from build123d import *

# Parameters (mm, degrees)
SKETCH1_R           = 9.2
BOSS_EXTRUDE1_DEPTH = 8.2
BOSS_EXTRUDE2_DEPTH = 1.8
LPATTERN1_COUNT     = 3
LPATTERN1_PITCH     = 20.2
FILLET1_R           = 1
CUT_EXTRUDE1_DEPTH  = 8.2


with BuildPart() as part:
    # Sketch1 → Boss-Extrude1 (new body)
    with BuildSketch(Plane(origin=(0, 0, 0), x_dir=(1, 0, 0), z_dir=(0, 1, 0))):
        Polygon((-9.1, 10.1), (-7, 10.1), (-7.5, 8.7), (-4.5, 8.7), (-5, 10.1), (5, 10.1), (4.5, 8.7), (7.5, 8.7), (7, 10.1), (9.1, 10.1), (10.1, 10.1), (10.1, 9.1), (10.1, 7), (10.1, 5), (10.1, -5), (10.1, -7), (10.1, -9.1), (10.1, -10.1), (9.1, -10.1), (7, -10.1), (7.5, -11.5), (4.5, -11.5), (5, -10.1), (-5, -10.1), (-4.5, -11.5), (-7.5, -11.5), (-7, -10.1), (-9.1, -10.1), (-10.1, -10.1), (-10.1, -9.1), (-10.1, -7), (-11.5, -7.5), (-11.5, -4.5), (-10.1, -5), (-10.1, 5), (-11.5, 4.5), (-11.5, 7.5), (-10.1, 7), (-10.1, 9.1), (-10.1, 10.1), align=None)
        with Locations(Location((0, 0, 0), (0, 0, 270))):
            Circle(SKETCH1_R, mode=Mode.SUBTRACT)
    boss_extrude1 = extrude(amount=BOSS_EXTRUDE1_DEPTH)

    # Sketch2 → Boss-Extrude2 (add)
    with BuildSketch(Plane(origin=(0, 8.2, 0), x_dir=(1, 0, 0), z_dir=(0, 1, 0))):
        with BuildLine():
            Line((-9.1, 4), (-5, 4))
            ThreePointArc((-5, 4), (-4.292893219, 4.292893219), (-4, 5))
            Line((-4, 5), (-4, 9.1))
            ThreePointArc((-4, 9.1), (-4.292893219, 9.807106781), (-5, 10.1))
            Line((-5, 10.1), (-9.1, 10.1))
            Line((-9.1, 10.1), (-10.1, 10.1))
            Line((-10.1, 10.1), (-10.1, 9.1))
            Line((-10.1, 9.1), (-10.1, 5))
            Line((-10.1, 5), (-10.1, 4))
            Line((-10.1, 4), (-9.1, 4))
        make_face()
        with BuildLine():
            Line((9.1, 10.1), (10.1, 10.1))
            Line((10.1, 10.1), (10.1, 4))
            Line((10.1, 4), (9.1, 4))
            Line((9.1, 4), (5, 4))
            ThreePointArc((5, 4), (4.292893219, 4.292893219), (4, 5))
            Line((4, 5), (4, 9.1))
            ThreePointArc((4, 9.1), (4.292893219, 9.807106781), (5, 10.1))
            Line((5, 10.1), (9.1, 10.1))
        make_face()
        with BuildLine():
            Line((9.1, -4), (5, -4))
            ThreePointArc((5, -4), (4.292893219, -4.292893219), (4, -5))
            Line((4, -5), (4, -9.1))
            ThreePointArc((4, -9.1), (4.292893219, -9.807106781), (5, -10.1))
            Line((5, -10.1), (9.1, -10.1))
            Line((9.1, -10.1), (10.1, -10.1))
            Line((10.1, -10.1), (10.1, -4))
            Line((10.1, -4), (9.1, -4))
        make_face()
        with BuildLine():
            Line((-4, -5), (-4, -9.1))
            ThreePointArc((-4, -9.1), (-4.292893219, -9.807106781), (-5, -10.1))
            Line((-5, -10.1), (-9.1, -10.1))
            Line((-9.1, -10.1), (-10.1, -10.1))
            Line((-10.1, -10.1), (-10.1, -9.1))
            Line((-10.1, -9.1), (-10.1, -5))
            Line((-10.1, -5), (-10.1, -4))
            Line((-10.1, -4), (-9.1, -4))
            Line((-9.1, -4), (-5, -4))
            ThreePointArc((-5, -4), (-4.292893219, -4.292893219), (-4, -5))
        make_face()
    boss_extrude2 = extrude(amount=BOSS_EXTRUDE2_DEPTH)

    # LPattern1: Boss-Extrude1, Boss-Extrude2 ×3
    with Locations(*[(i * LPATTERN1_PITCH, 0, 0) for i in range(1, LPATTERN1_COUNT)]):
        add(boss_extrude1)
        add(boss_extrude2)

    # Fillet1
    fillet1_edges = [part.edges().sort_by_distance(p)[0] for p in [
        (50.5, 5, 10.1),
        (50.5, 5, -10.1),
        (-10.1, 5, 10.1),
        (-10.1, 5, -10.1),
    ]]
    fillet(fillet1_edges, radius=FILLET1_R)

    # Sketch5 → Cut-Extrude1 (cut)
    with BuildSketch(Plane.XZ):
        Polygon((50.5, -5), (49.1, -4.5), (49.1, -7.5), (50.5, -7), align=None)
    cut_extrude1 = extrude(amount=-CUT_EXTRUDE1_DEPTH, mode=Mode.SUBTRACT)

    # Mirror1: Cut-Extrude1 across plane
    add(cut_extrude1.mirror(Plane.XY), mode=Mode.SUBTRACT)


solid = part.part
Verification items for the finished model (mm, model axes). A direction names the side the tool comes from. Coordinates: 2 decimals unless noted, no trailing zeros. Order: outer loops, then holes, each group sorted by start corner. A loop starts at its lowest first (then second) coordinate and runs counter-clockwise, first axis right, second up. Notation, with made-up numbers: (53.5, 17.25) -> (89.5, 17.25) arc R6 cw to (89.5, 26.25) -> close; hole circle Ø4 at (26, -17.5). An arc over 180 degrees is marked (long way). Put each result on its own line as item: value. Start each with the question number.
1. Cross-section at C-C, the plane y = 9. Count the separate pieces of the cut face and the enclosed holes in it, then the cut area to 3 significant figures.
2. Material ranges on L1, parallel to X at y = 4, z = 0; L2, parallel to X at y = 8.75, z = -9; L3, parallel to Z at x = 40.4, y = 3.5, recorded low to high. Write a range as [from, to].
3. Access from +Z, -Z, +X, -X, +Y, -Y to the whole of each face (thin tool, end or side, straight path). Record for faces 5 (the flat face through (-6, 8.2, 11)), 6 (the cylindrical face through (44.701, 9.087, 4.285)), 7 (the flat face through (-6, 8.2, 6)), 8 (the flat face through (24.2, 9, 7)), 9 (the flat face through (47.646, 4.043, 10.79)).
4. Cross-section at B-B, the plane x = 0. Record the boundary of the cut face in (y, z).
5. Go/stop test with flat-tipped pins: pin 1 Ø1.8 at (x, z) = (29.5, -2) entering from +Y; pin 2 Ø2 at (x, z) = (43, -3.5) entering from -Y; pin 3 Ø0.5 at (y, z) = (9, 7) entering from -X; pin 4 Ø1.5 at (x, y) = (-1.5, 8) entering from +Z. Record where each tip stops, or that it passes through.
6. Cross-section at D-D, the plane x = 38.5. Record the boundary of the cut face in (y, z).
7. Mould release check, pull along Z, two halves, no side actions. Record for faces 1 (the flat face through (-8, 9, -4)), 2 (the cylindrical face through (36.115, 9.087, 9.799)), 3 (the flat face through (30, 10, -7)), 4 (the flat face through (-7.5, 6, -10.1)): released by +Z, released by -Z, zero draft, split by the parting line, or undercut.
8. Cross-section at A-A, the plane z = 0. Record the boundary of the cut face in (x, y).
Computed:
1. separate pieces: 8
1. enclosed holes: 0
1. area: 441 mm2
2. L1: [-10.1, -9.2], [9.2, 11], [29.4, 31.2], [49.6, 50.5]
2. L2: [-10.1, -4], [4, 16.2], [24.2, 36.4], [44.4, 50.5]
2. L3: [-10.1, -9.2], [9.2, 10.1]
3. face 5: +Z, +X, -X, +Y
3. face 6: +Y, -Y
3. face 7: -Y
3. face 8: +Z, -Z, +Y
3. face 9: +X, +Y, -Y
4. outline: (0, -10.1) -> (8.2, -10.1) -> (8.2, -9.2) -> (0, -9.2) -> close; (0, 9.2) -> (8.2, 9.2) -> (8.2, 10.1) -> (0, 10.1) -> close
5. pin 1: y = 8.2
5. pin 2: through
5. pin 3: x = -10.1
5. pin 4: z = 10.1
6. outline: (0, -10.1) -> (8.2, -10.1) -> (8.2, -9) -> (0, -9) -> close; (0, 9) -> (8.2, 9) -> (8.2, 10.1) -> (0, 10.1) -> close
7. face 1: undercut
7. face 2: released by +Z
7. face 3: zero draft
7. face 4: released by -Z
8. outline: (-10.1, 0) -> (-9.2, 0) -> (-9.2, 8.2) -> (-10.1, 8.2) -> close; (9.2, 0) -> (11, 0) -> (11, 8.2) -> (9.2, 8.2) -> close; (29.4, 0) -> (31.2, 0) -> (31.2, 8.2) -> (29.4, 8.2) -> close; (49.6, 0) -> (50.5, 0) -> (50.5, 8.2) -> (49.6, 8.2) -> close
